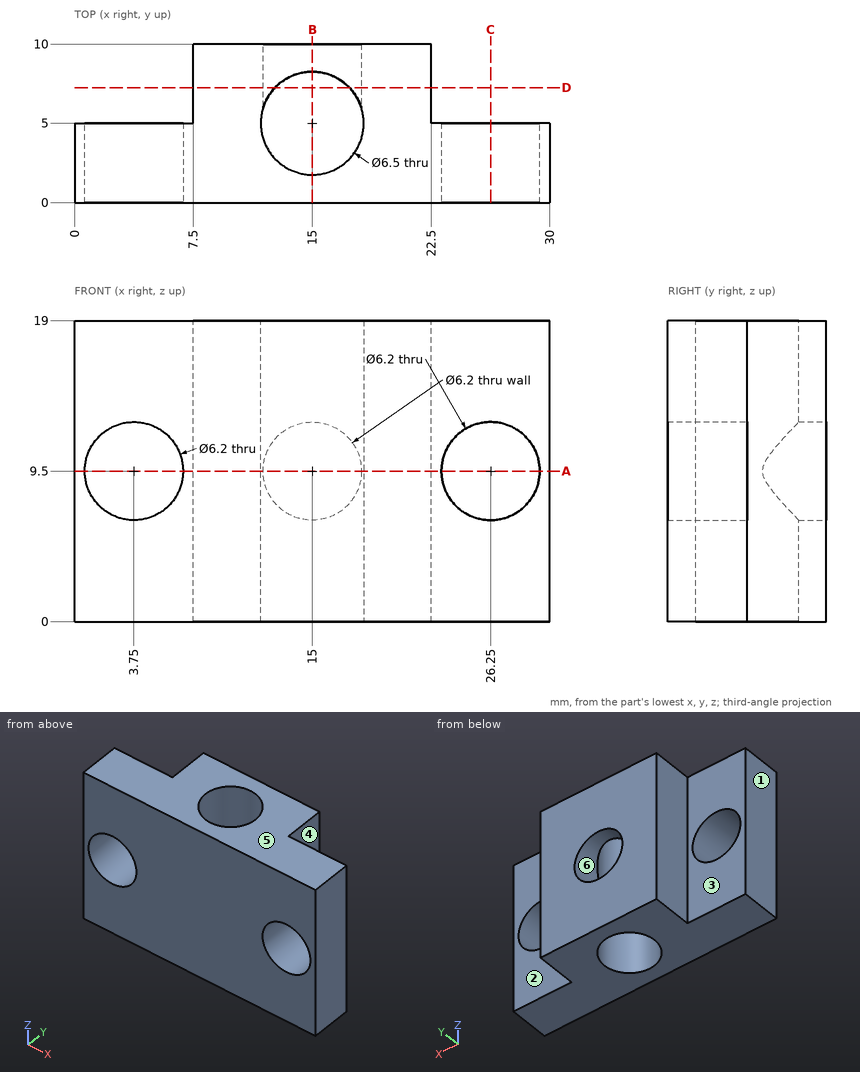
Verification items for this drawing (mm, ordinates from the low corner). A direction names the side the tool comes from. Give positions to 0.01 mm unless a question says otherwise; leave off trailing zeros. Loops run counter-clockwise (first coordinate to the right, second up) from the corner with the lowest first, then second, coordinate; pieces in that order, holes last. Notation, with made-up numbers: M 51.25,47 L 56.25,47 A10 ccw 56.25,63 Z; hole C 73.5,72.25 d8. An arc over 180 degrees is marked long. Write item = value, one per line. Start each with the question number.
1. Section check B-B, the plane x = 15. Enter the section's corners in (y, z).
2. Tool access check on the marked faces 1, 2 and 3. Record the directions out of +Z, -Z, +X, -X, +Y, -Y that give a thin tool (end or side, any length) a straight path to the whole face; none if there is none.
3. Section check C-C, the plane x = 26.25. Enter the section's corners in (y, z).
4. Section check A-A, the plane z = 9.5. Enter the section's corners in (x, y).
5. Section check D-D, the plane y = 7.25. Enter the section's corners in (x, z), plus the area to 3 significant figures.
6. Thickness scan on probe 1 along Z at (x, y) = (3.75, 3.85); probe 2 along X at (y, z) = (4, 7.5); probe 3 along X at (y, z) = (2.25, 9.25). Record the ranges inside material, lowest first.
7. Go/stop test with flat-tipped pins: P1, Ø10, axis at x = 3.75, z = 9.5, coming from the +Y side; P2, Ø2, axis at x = 28, z = 11.5, coming from the +Y side; P3, Ø5.5, axis at x = 15, z = 9.5, coming from the +Y side; P4, Ø5, axis at y = 8, z = 10, coming from the +X side. Record where each tip stops, or that it passes through.
8. Draft check along Z on the marked faces 4, 5 and 6. Enter one of: +Z half, -Z half, draft (parallel to the pull), parting line (faces both ways), or undercut.
Values follow:
q1.outline = M 0,0 L 1.75,0 L 1.75,19 L 0,19 Z; M 8.25,0 L 10,0 L 10,6.4 L 8.25,6.4 Z; M 8.25,12.6 L 10,12.6 L 10,19 L 8.25,19 Z
q2.face_1 = +Z, -Z, -X, +Y, -Y
q2.face_2 = +Z, -Z, +X, +Y
q2.face_3 = +Z, -Z, -X, +Y
q3.outline = M 0,0 L 5,0 L 5,6.4 L 0,6.4 Z; M 0,12.6 L 5,12.6 L 5,19 L 0,19 Z
q4.outline = M 0,0 L 0.65,0 L 0.65,5 L 0,5 Z; M 6.85,0 L 23.15,0 L 23.15,5 L 22.5,5 L 22.5,10 L 18.1,10 L 18.1,5.98 A3.25 cw long 11.9,5.98 L 11.9,10 L 7.5,10 L 7.5,5 L 6.85,5 Z; M 29.35,0 L 30,0 L 30,5 L 29.35,5 Z
q5.outline = M 7.5,0 L 12.65,0 L 12.65,7.47 A3.1 cw 12.65,11.53 L 12.65,19 L 7.5,19 Z; M 17.35,0 L 22.5,0 L 22.5,19 L 17.35,19 L 17.35,11.53 A3.1 cw 17.35,7.47 Z
q5.area = 192 mm^2
q6.probe_1 = 0 to 6.4, 12.6 to 19
q6.probe_2 = 0 to 1.38, 6.12 to 11.91, 18.09 to 23.88, 28.62 to 30
q6.probe_3 = 0 to 0.66, 6.84 to 13.27, 16.73 to 23.16, 29.34 to 30
q7.P1 = 10
q7.P2 = 5
q7.P3 = 3.27
q7.P4 = 22.5
q8.face_4 = draft
q8.face_5 = +Z half
q8.face_6 = undercut
